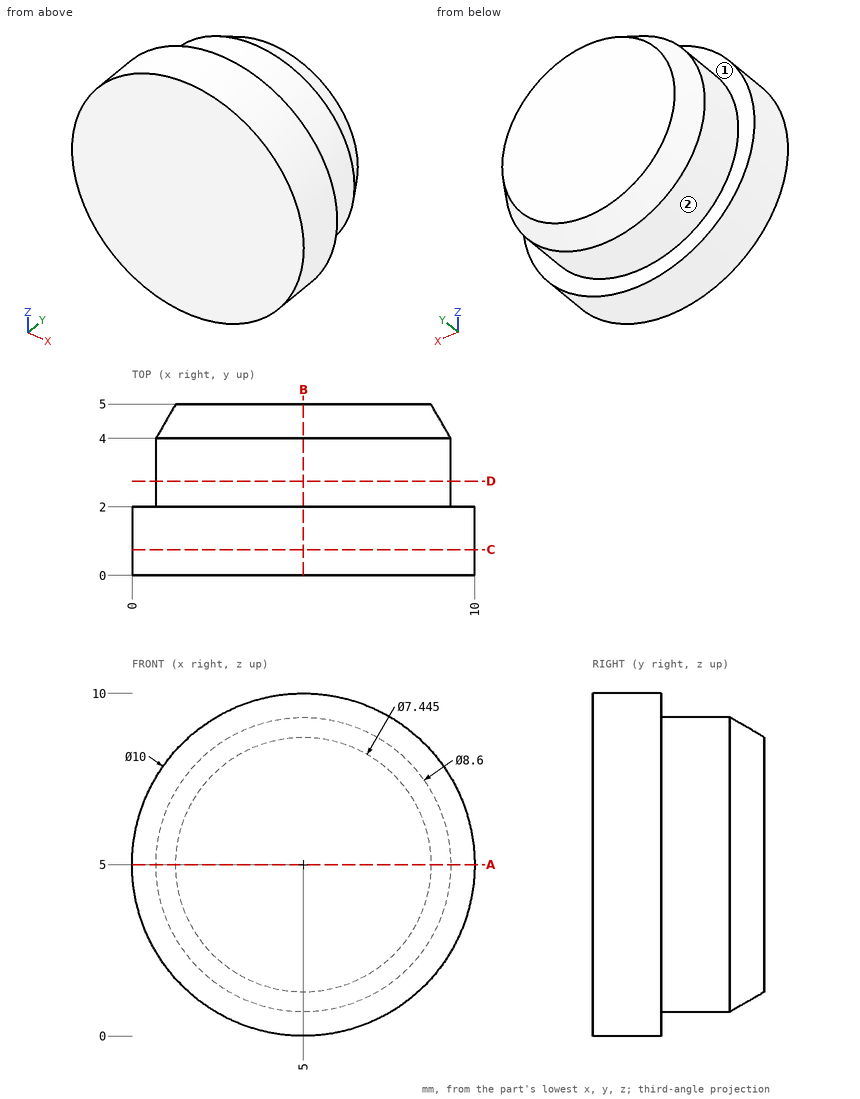
Could you check a few things on this drawing? It's one solid part, dimensions in mm from its lowest x, y, z. Coordinates: 2 decimals unless noted, no trailing zeros. Order: outer loops, then holes, each group sorted by start corner. A loop starts at its lowest first (then second) coordinate and runs counter-clockwise, first axis right, second up. Notation, with made-up numbers: (36, -14) - (69, -14) arc R25 cw to (69, 24) - close; hole circle Ø6 at (57.5, 44.5). An arc over 180 degrees is marked (long way). One line per question, with ' | ' between items.
(1) If I drill on L1, parallel to Y at x = 8.5, z = 8.5; L2, parallel to X at y = 3, z = 5; L3, parallel to Z at x = 4, y = 2.35, over which ranges is the centre line in solid material (lowest first)?
Report:
L1: y = 0 to 2 | L2: x = 0.7 to 9.3 | L3: z = 0.82 to 9.18
(2) Suppose I cut it at C-C on y = 0.75. List the corners of the cut face in (x, z) for me.
Report:
outline: circle Ø10 at (5, 5)
(3) If we mould it in two halves opening along X, with no side actions, what happens to the marked faces 1 and 2? For each: pulls with the +X half, pulls with the -X half, needs draft (parallel to the pull), parting line crosses it, or undercut.
Report:
face 1: needs draft | face 2: parting line crosses it
(4) Suppose I cut it at D-D on y = 2.75. List the corners of the cut face in (x, z) for me.
Report:
outline: circle Ø8.6 at (5, 5)
(5) Suppose I cut it at B-B on x = 5. List the corners of the cut face in (y, z) for me, and give its area (3 significant figures).
Report:
outline: (0, 0) - (2, 0) - (2, 0.7) - (4, 0.7) - (5, 1.28) - (5, 8.72) - (4, 9.3) - (2, 9.3) - (2, 10) - (0, 10) - close | area: 45.2 mm2
(6) Suppose I cut it at A-A on z = 5. List the corners of the cut face in (x, y) for me.
Report:
outline: (0, 0) - (10, 0) - (10, 2) - (9.3, 2) - (9.3, 4) - (8.72, 5) - (1.28, 5) - (0.7, 4) - (0.7, 2) - (0, 2) - close
